Design review of the part built by this model. Coordinates are the model's own, in mm. Face numbers are marked on the shaded views. A direction names the side the tool comes from. Coordinates: 2 decimals unless noted, no trailing zeros. Loops run counter-clockwise (first coordinate to the right, second up) from the corner with the lowest first, then second, coordinate; pieces in that order, holes last. Notation, with made-up numbers: (38.5, 13.25) -> (92.5, 13.25) arc R28 cw to (92.5, 32.25) -> close; hole circle Ø7 at (21.5, 78.25). An arc over 180 degrees is marked (long way). Answer as a JSON object with one key per item and string values.
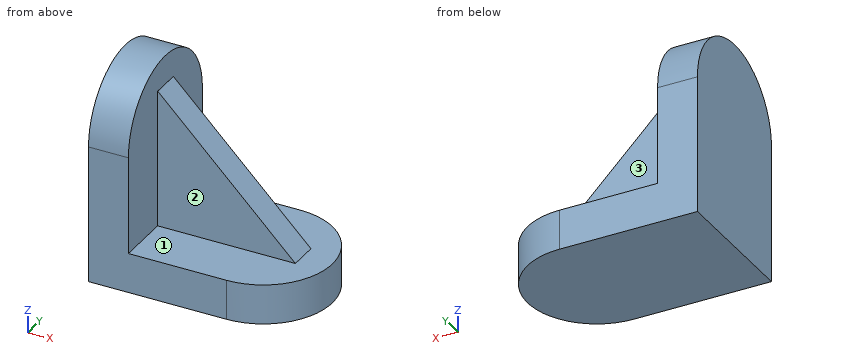
```python
from build123d import *

# Parameters (mm, degrees)
F1_W     = 38
F1_H     = 38
F2_DEPTH = 11
F3_DEPTH = 11
F9_E8_W  = 53.7300702473
F9_E8_H  = 8


with BuildPart() as f2:
    # F1 (on Right) → F2 (new body)
    with BuildSketch(Plane.YZ):
        with Locations((19, 19)):
            Rectangle(F1_W, F1_H)
        with BuildLine():
            ThreePointArc((38, 38), (19, 57), (0, 38))
            Line((0, 38), (38, 38))
        make_face()
    extrude(amount=F2_DEPTH)

    # F0 (on Top) → F3 (join)
    with BuildSketch(Plane.XY):
        with BuildLine():
            Line((0, 38), (0, 0))
            Line((0, 0), (38, 0))
            ThreePointArc((38, 0), (57, 19), (38, 38))
            Line((38, 38), (0, 38))
        make_face()
    extrude(amount=F3_DEPTH)

    # F9_E8 (on explicit) → F10 (join, up to the next surface of F2)
    with BuildSketch(Plane(origin=(11.0387885943, 23, 49), x_dir=(0.7065170626, 0, -0.7076960083), z_dir=(-0.7076960083, 0, -0.7065170626))):
        with Locations((26.8650351237, 4)):
            Rectangle(F9_E8_W, F9_E8_H)
    extrude(until=Until.NEXT)


solid = f2.part
```
1) Clearance check with flat-ended pins moving along their axes: pin 1 Ø2 at (x, y) = (20, 31.5) entering from -Z; pin 2 Ø6 at (x, y) = (41.5, 25) entering from +Z; pin 3 Ø19 at (x, z) = (26, 39.5) entering from +Y; pin 4 Ø11.5 at (y, z) = (20.5, 36.5) entering from +X. State where each tip first meets the part, or that it passes through.
Completed:
{"pin 1": "z = 0", "pin 2": "z = 20.73", "pin 3": "y = 23", "pin 4": "x = 29.26"}
2) Add section A-A, the plane y = 19. Give the boundary of the cut face in (x, z).
Completed:
{"outline": "(0, 0) -> (57, 0) -> (57, 11) -> (48.98, 11) -> (11.04, 49) -> (11, 48.96) -> (11, 57) -> (0, 57) -> close"}
3) Add section D-D, the plane x = 7. Give the boundary of the cut face in (y, z).
Completed:
{"outline": "(0, 0) -> (38, 0) -> (38, 38) arc R19 ccw to (0, 38) -> close"}
4) Add section B-B, the plane x = 14.5. Give the boundary of the cut face in (y, z), and give its area (3 significant figures).
Completed:
{"outline": "(0, 0) -> (38, 0) -> (38, 11) -> (23, 11) -> (23, 45.53) -> (15, 45.53) -> (15, 11) -> (0, 11) -> close", "area": "694 mm²"}
5) For the marked faces 1, 2 and 3, list the 3-axis set-ups (+Z, -Z, +X, -X, +Y, -Y) from which the entire face can be reached by the end or side of a thin tool; tool diameter is ignored.
Completed:
{"face 1": "+Z, +X", "face 2": "+Z, +X, -Y", "face 3": "+Z, +X, +Y"}
6) Add section C-C, the plane z = 52.5. Give the boundary of the cut face in (x, y).
Completed:
{"outline": "(0, 6.72) -> (11, 6.72) -> (11, 31.28) -> (0, 31.28) -> close"}
7) Wall thickness on probe 1 along X at (y, z) = (26.5, 44.5); probe 2 along Y at (x, z) = (35.5, 19.5): over which ranges is each line inside the solid? List them lowest first.
Completed:
{"probe 1": "0 to 11", "probe 2": "15 to 23"}
